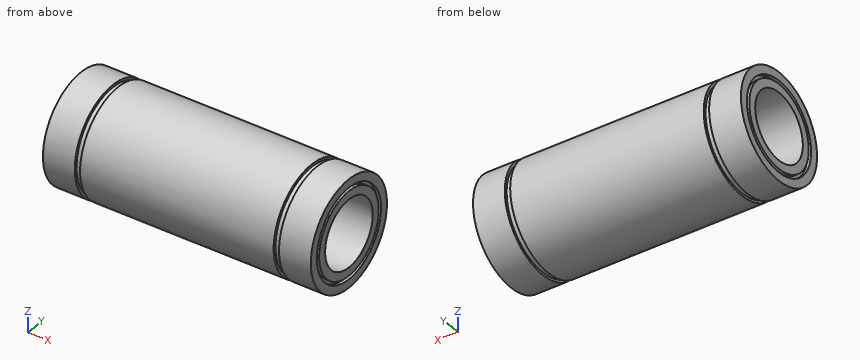
from build123d import *


with BuildPart() as part:
    # Esboço1 → Revolução1 (revolve)
    with BuildSketch(Plane.XY):
        Polygon((-40, 16), (-30.5, 16), (-30.5, 15.25), (-28.9, 15.25), (-28.9, 16), (28.9, 16), (28.9, 15.25), (30.5, 15.25), (30.5, 16), (40, 16), (40, 13.5), (39, 13.5), (39, 12.5), (40, 12.5), (40, 10), (-40, 10), (-40, 12.5), (-39, 12.5), (-39, 13.5), (-40, 13.5), align=None)
    revolve(axis=Axis((0, 0, 0), (-1, 0, 0)))


solid = part.part
Input: part model. Units: mm. Frame: model coordinates. Give positions to 0.01 mm unless a question says otherwise; leave off trailing zeros. Order: outer loops, then holes, each group sorted by start corner. A loop starts at its lowest first (then second) coordinate and runs counter-clockwise, first axis right, second up.
Q1. Contact query for flat-ended pins moving along their axis: pin 1 Ø5 at (x, y) = (-25, -8) entering from +Z (3 decimals); pin 2 Ø4 at (x, y) = (12.5, -9.5) entering from +Z; pin 3 Ø2 at (x, y) = (28.5, 12) entering from +Z. Output: stop coordinate, or through.
Checked values:
pin 1: stops at z = 15.025
pin 2: stops at z = 14.13
pin 3: stops at z = 11.62
Q2. Section A-A on x = -15.5. Output: boundary loops of the cut face in (y, z), and give its area (3 significant figures).
Checked values:
outline: circle Ø32 at (0, 0); hole circle Ø20 at (0, 0)
area: 490 mm2
Q3. Ray query, probe 1 along Z at (x, y) = (39.8, 0); probe 2 along Z at (x, y) = (-13, 0). Return the intervals inside material, ascending.
Checked values:
probe 1: z = -16 to -13.5, -12.5 to -10, 10 to 12.5, 13.5 to 16
probe 2: z = -16 to -10, 10 to 16
